```python
from build123d import *

# Parameters (mm, degrees)
PAD_DEPTH = 80


with BuildPart() as part:
    # Sketch → Pad (new body)
    with BuildSketch(Plane.XY):
        with BuildLine():
            Line((-53.441865, 0), (46.558135, 0))
            ThreePointArc((54.558135, -8), (52.214989, -2.343146), (46.558135, 0))
            Line((54.558135, -58), (54.558135, -8))
            Line((64.558135, -58), (54.558135, -58))
            Line((64.558135, -48), (64.558135, -58))
            ThreePointArc((66.558135, -48), (65.558135, -47), (64.558135, -48))
            Line((66.558135, -60), (66.558135, -48))
            ThreePointArc((52.558135, -60), (59.558135, -67), (66.558135, -60))
            Line((52.558135, -8), (52.558135, -60))
            ThreePointArc((52.558135, -8), (50.800776, -3.757359), (46.558135, -2))
            Line((-55.441865, -2), (46.558135, -2))
            ThreePointArc((-55.441865, 12), (-62.441865, 5), (-55.441865, -2))
            Line((-43.441865, 12), (-55.441865, 12))
            ThreePointArc((-43.441865, 10), (-42.441865, 11), (-43.441865, 12))
            Line((-53.441865, 10), (-43.441865, 10))
            Line((-53.441865, 0), (-53.441865, 10))
        make_face()
    extrude(amount=PAD_DEPTH)


solid = part.part
```
Could you check a few things on this model? Use its own coordinates, in mm. A direction names the side the tool comes from. Coordinates: 2 decimals unless noted, no trailing zeros. Write each loop counter-clockwise with the first axis right and the second up, starting at its lowest first coordinate (ties: lowest second). Pieces come first, ordered by that corner, then holes. Notation, with made-up numbers: M 63,-38.5 L 70,-38.5 A26 cw 70,-17.5 Z; hole C 46.5,-35.5 d5. An arc over 180 degrees is marked long. Answer as CSV lines item,"result". Start each with the question number.
1) We'd pull the mould along Y, two halves only. Please class faces 4 (the flat face through (-49, 12, 39)), 5 (the flat face through (-49, 10, 39)), 6 (the flat face through (-5, -2, 39)), 7 (the flat face through (-53.442, 5, 39)): +Y half, -Y half, draft (parallel to the pull), parting line (faces both ways), or undercut.
2) I want a section at A-A, the plane z = 6.5. Please give me the cut outline in (x, y), and give its area (3 significant figures).
3) For P1, Ø11, axis at y = -51.5, z = 54.5, coming from the -X side; P2, Ø1, axis at x = -0.5, z = 60, coming from the -Y side; P3, Ø4, axis at y = -1, z = 49, coming from the -X side, each with a flat end and sliding along its axis, tell me the tip position at first contact or that it passes through.
4) I want a section at B-B, the plane y = 5. Please give me the cut outline in (x, z).
5) I want a section at C-C, the plane x = -36. Please give me the cut outline in (y, z).
6) Please list where these lines run through material, in increasing order: line 1 (Y direction, x = -45.5, z = 74.5); line 2 (X direction, y = -32, z = 66); line 3 (Y direction, x = 32.5, z = 68.5). Write a range as from..to.
7) For faces 1 (the cylindrical face through (59.4, -67, 39.4)), 2 (the flat face through (54.558, -33, 39)), 3 (the flat face through (52.558, -34, 39)), which set-ups out of +Z, -Z, +X, -X, +Y, -Y let a thin tool reach every point of the face, with its end or its side?
Data:
1,face 4,"+Y half"
1,face 5,"undercut"
1,face 6,"-Y half"
1,face 7,"undercut"
2,outline,"M -55.44,-2 L 46.56,-2 A6 cw 52.56,-8 L 52.56,-60 A7 ccw 66.56,-60 L 66.56,-48 A1 ccw 64.56,-48 L 64.56,-58 L 54.56,-58 L 54.56,-8 A8 ccw 46.56,0 L -53.44,0 L -53.44,10 L -43.44,10 A1 ccw -43.44,12 L -55.44,12 A7 ccw Z"
2,area,"575 mm^2"
3,P1,"stops at x = 52.56"
3,P2,"stops at y = -2"
3,P3,"stops at x = -61.19"
4,outline,"M -62.44,0 L -53.44,0 L -53.44,80 L -62.44,80 Z"
5,outline,"M -2,0 L 0,0 L 0,80 L -2,80 Z"
6,line 1,"y = -2..0, 10..12"
6,line 2,"x = 52.56..54.56"
6,line 3,"y = -2..0"
7,face 1,"+Z, -Z, -Y"
7,face 2,"+Z, -Z, +Y"
7,face 3,"+Z, -Z, -X, -Y"
